The drawing under review shows one solid part. Ordinate dimensions are in mm from its lowest x, y, z. Coordinates: 2 decimals unless noted, no trailing zeros. Order: outer loops, then holes, each group sorted by start corner. A loop starts at its lowest first (then second) coordinate and runs counter-clockwise, first axis right, second up.
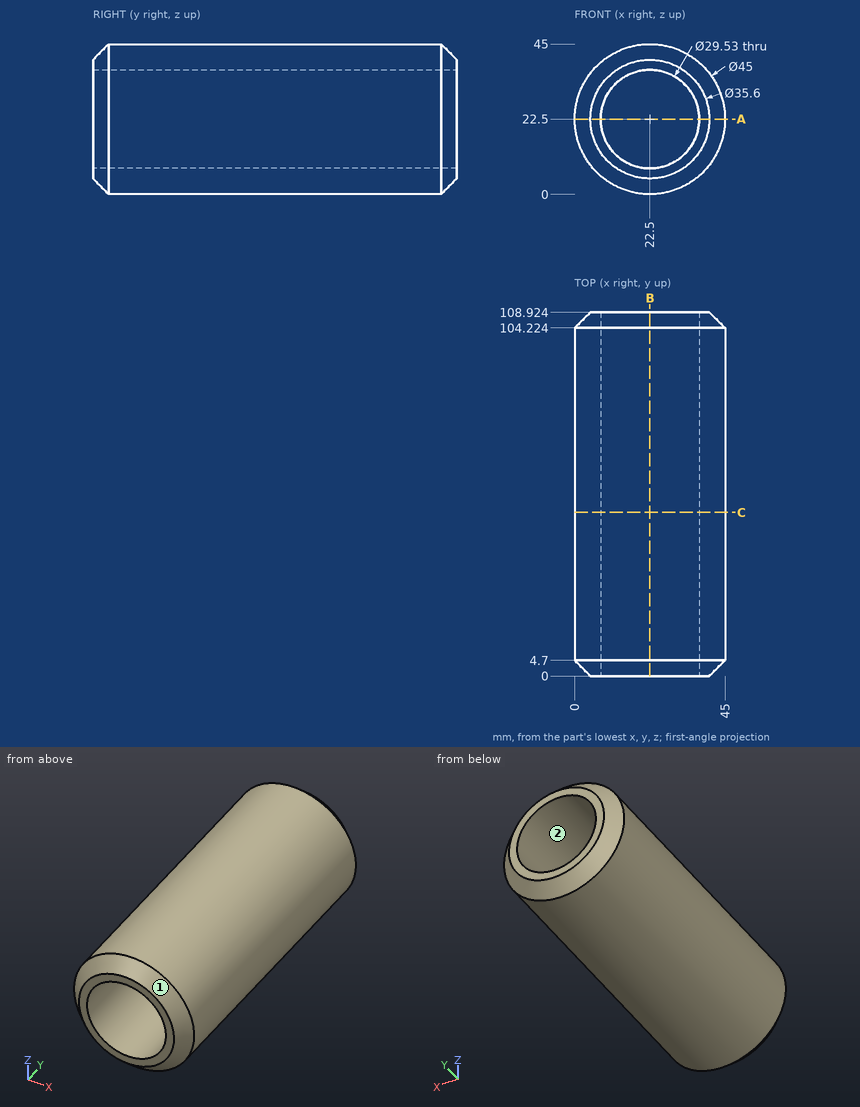
(1) We need section C-C, the plane y = 49. Write out the cut boundary in (x, z) (1 decimal).
A:
outline: circle Ø45 at (22.5, 22.5); hole circle Ø29.5 at (22.5, 22.5)
(2) We need section A-A, the plane z = 22.5. Write out the cut boundary in (x, y) (1 decimal).
A:
outline: (0, 4.7) - (4.7, 0) - (7.7, 0) - (7.7, 108.9) - (4.7, 108.9) - (0, 104.2) - close; (37.3, 0) - (40.3, 0) - (45, 4.7) - (45, 104.2) - (40.3, 108.9) - (37.3, 108.9) - close
(3) Draft analysis for pull direction Z (two halves, no side actions). For the marked faces 1 and 2, state which applies: released by +Z, released by -Z, zero draft, split by the parting line, or undercut.
A:
face 1: split by the parting line
face 2: undercut
(4) Wall thickness on probe 1 along X at (y, z) = (57, 22) (1 decimal); probe 2 along Z at (x, y) = (34, 24.5): over which ranges is each line inside the solid? List them lowest first.
A:
probe 1: x = 0 to 7.7, 37.3 to 45
probe 2: z = 3.16 to 13.24, 31.76 to 41.84
(5) For pin 1 Ø10 at (y, z) = (97.5, 19) entering from +X; pin 2 Ø8 at (x, z) = (38, 6.5) entering from -Y (1 decimal); pin 3 Ø3 at (x, y) = (30.5, 47) entering from +Z; pin 4 Ø2 at (x, z) = (39, 5.5) entering from -Y, all flat-tipped, find the tip position at first contact; note any pin that passes through.
A:
pin 1: stops at x = 45
pin 2: stops at y = 0.5
pin 3: stops at z = 44.04
pin 4: passes through
(6) We need section B-B, the plane x = 22.5. Write out the cut boundary in (y, z) (1 decimal).
A:
outline: (0, 4.7) - (4.7, 0) - (104.2, 0) - (108.9, 4.7) - (108.9, 7.7) - (0, 7.7) - close; (0, 37.3) - (108.9, 37.3) - (108.9, 40.3) - (104.2, 45) - (4.7, 45) - (0, 40.3) - close
